Check sheet for the modelled part. Datum: model origin and axes. Units: mm. Face numbers are marked on the shaded views. Give positions to 0.01 mm unless a question says otherwise; leave off trailing zeros. Write each loop counter-clockwise with the first axis right and the second up, starting at its lowest first coordinate (ties: lowest second). Pieces come first, ordered by that corner, then holes. Notation, with made-up numbers: (89, 1.5) -> (130, 1.5) arc R4 cw to (130, 8.5) -> close; hole circle Ø9 at (0.5, 68.25). An arc over 180 degrees is marked (long way). Use a Markdown table: item, result. Add a question column.
1. Scan lines: probe 1 along X at (y, z) = (-58.5, 0.25); probe 2 along Z at (x, y) = (20, -7.5); probe 3 along X at (y, z) = (-11, 4). Record each from-to range of solid material in increasing order. Write a range as [from, to].
2. Release check for a two-part mould opening along X. For the marked faces 1, 2 and 3 record: released by +X, released by -X, zero draft, split by the parting line, or undercut.
3. Cross-section at C-C (z = 2.5). Enter the section's corners in (x, y), then the cut area to 3 significant figures.
4. Cross-section at A-A (x = 0). Enter the section's corners in (y, z), then the cut area to 3 significant figures.
5. Cross-section at B-B (y = 52). Enter the section's corners in (x, z), then the cut area to 3 significant figures.
6. Gauge pin test, flat end, axial feed: P1, Ø2, axis at x = 4, z = 2.5, coming from the +Y side. Record the tip position at first contact, or that the pin passes through.
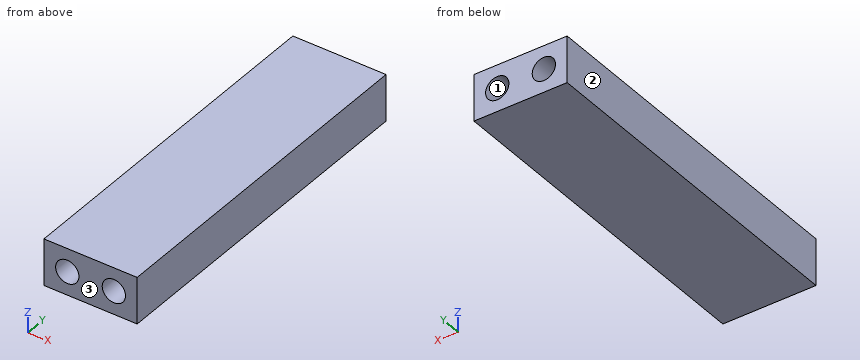
from build123d import *

# Parameters (mm, degrees)
F0_R          = 5
F1_DEPTH      = 75
F1_DEPTH_BACK = 75


with BuildPart() as f1:
    # F0 (on Front) → F1 (new body, two sides)
    with BuildSketch(Plane.XZ) as f1_sk:
        Polygon((-10, -10), (10, -10), (30, -10), (30, 10), (10, 10), (-10, 10), align=None)
        Circle(F0_R, mode=Mode.SUBTRACT)
        with Locations((20, 0)):
            Circle(F0_R, mode=Mode.SUBTRACT)
    extrude(amount=F1_DEPTH)
    extrude(f1_sk.sketch, amount=-F1_DEPTH_BACK)


solid = f1.part
Worked answers:
| question | item | result |
|---|---|---|
| 1 | probe 1 | x = [-10, -4.99], [4.99, 15.01], [24.99, 30] |
| 1 | probe 2 | z = [-10, -5], [5, 10] |
| 1 | probe 3 | x = [-10, -3], [3, 17], [23, 30] |
| 2 | face 1 | undercut |
| 2 | face 2 | released by -X |
| 2 | face 3 | zero draft |
| 3 | outline | (-10, -75) -> (-4.33, -75) -> (-4.33, 75) -> (-10, 75) -> close; (4.33, -75) -> (15.67, -75) -> (15.67, 75) -> (4.33, 75) -> close; (24.33, -75) -> (30, -75) -> (30, 75) -> (24.33, 75) -> close |
| 3 | area | 3,400 mm² |
| 4 | outline | (-75, -10) -> (75, -10) -> (75, -5) -> (-75, -5) -> close; (-75, 5) -> (75, 5) -> (75, 10) -> (-75, 10) -> close |
| 4 | area | 1,500 mm² |
| 5 | outline | (-10, -10) -> (30, -10) -> (30, 10) -> (-10, 10) -> close; hole circle Ø10 at (0, 0); hole circle Ø10 at (20, 0) |
| 5 | area | 643 mm² |
| 6 | P1 | stops at y = 75 |
